from build123d import *

# Parameters (mm, degrees)
CROQUIS1_R              = 100
SALIENTE_EXTRUIR1_DEPTH = 3
CROQUIS3_R              = 110
CORTAR_EXTRUIR1_DEPTH   = 3
REDONDEO1_R             = 10
CORTAR_EXTRUIR2_DEPTH   = 142.453172607
CROQUIS6_W              = 10
CROQUIS6_H              = 50
CROQUIS6_W_2            = 30
CROQUIS6_H_2            = 10
CORTAR_EXTRUIR4_DEPTH   = 10
REDONDEO3_R             = 5
CROQUIS7_R              = 1.5
CORTAR_EXTRUIR5_DEPTH   = 142.453172607
CROQUIS8_R              = 1.5
CORTAR_EXTRUIR6_DEPTH   = 142.453172607
CROQUIS9_R              = 2
CORTAR_EXTRUIR7_DEPTH   = 142.453172607


with BuildPart() as part:
    # Croquis1 → Saliente-Extruir1 (new body)
    with BuildSketch(Plane.XY):
        Circle(CROQUIS1_R)
    extrude(amount=SALIENTE_EXTRUIR1_DEPTH)

    # Croquis3 → Cortar-Extruir1 (cut)
    with BuildSketch(Plane.XY.offset(3)):
        with Locations((190, 0)):
            Circle(CROQUIS3_R)
    extrude(amount=-CORTAR_EXTRUIR1_DEPTH, mode=Mode.SUBTRACT)

    # Redondeo1
    redondeo1_edges = [part.edges().sort_by_distance(p)[0] for p in [
        (89.473684211, -44.659375654, 1.5),
        (89.473684211, 44.659375654, 1.5),
    ]]
    fillet(redondeo1_edges, radius=REDONDEO1_R)

    # Croquis4 → Cortar-Extruir2 (cut, through all)
    with BuildSketch(Plane.XY.offset(3)):
        Polygon((-57.629202667, -83.792153571), (-83.792153571, -57.629202667), (-68.235804385, -42.072853481), (-42.072853481, -68.235804385), align=None)
        Polygon((-57.629202667, 83.792153571), (-42.072853481, 68.235804385), (-68.235804385, 42.072853481), (-83.792153571, 57.629202667), align=None)
        Polygon((83.792153571, 57.629202667), (68.235804385, 42.072853481), (42.072853481, 68.235804385), (57.629202667, 83.792153571), align=None)
        Polygon((57.629202667, -83.792153571), (42.072853481, -68.235804385), (68.235804385, -42.072853481), (83.792153571, -57.629202667), align=None)
    extrude(amount=-CORTAR_EXTRUIR2_DEPTH, mode=Mode.SUBTRACT)

    # Croquis6 → Cortar-Extruir4 (cut)
    with BuildSketch(Plane.XY.offset(3)):
        with Locations((-68.235804385, 0)):
            Rectangle(CROQUIS6_W, CROQUIS6_H)
        with Locations((0, 73.24)):
            Rectangle(CROQUIS6_W_2, CROQUIS6_H_2)
        with Locations((0, -73.24)):
            Rectangle(CROQUIS6_W_2, CROQUIS6_H_2)
    extrude(amount=-CORTAR_EXTRUIR4_DEPTH, mode=Mode.SUBTRACT)

    # Redondeo3
    redondeo3_edges = [part.edges().sort_by_distance(p)[0] for p in [
        (15, -78.24, 1.5),
        (-15, -78.24, 1.5),
        (15, -68.24, 1.5),
        (-15, -68.24, 1.5),
        (-73.235804385, -25, 1.5),
        (-63.235804385, -25, 1.5),
        (-73.235804385, 25, 1.5),
        (-63.235804385, 25, 1.5),
        (-15, 68.24, 1.5),
        (15, 68.24, 1.5),
        (-15, 78.24, 1.5),
        (15, 78.24, 1.5),
    ]]
    fillet(redondeo3_edges, radius=REDONDEO3_R - 0.0001)  # a hair under: the kernel refuses the full size

    # Croquis7 → Cortar-Extruir5 (cut, through all)
    with BuildSketch(Plane(origin=(0, 0, 0), x_dir=(-1, 0, 0), z_dir=(0, 0, -1))):
        with Locations((37.565, -24.17)):
            Circle(CROQUIS7_R)
        with Locations((-37.565, -24.17)):
            Circle(CROQUIS7_R)
        with Locations((-45.065, 24.17)):
            Circle(CROQUIS7_R)
        with Locations((37.565, 24.17)):
            Circle(CROQUIS7_R)
        with Locations((-14.06559482, 19.297497716)):
            Circle(CROQUIS7_R)
        with Locations((-14.061195262, -8.714642909)):
            Circle(CROQUIS7_R)
    extrude(amount=-CORTAR_EXTRUIR5_DEPTH, mode=Mode.SUBTRACT)

    # Croquis8 → Cortar-Extruir6 (cut, through all)
    with BuildSketch(Plane(origin=(0, 0, 0), x_dir=(-1, 0, 0), z_dir=(0, 0, -1))):
        with Locations((-20.32, 35)):
            Circle(CROQUIS8_R)
        with Locations((20.32, 35)):
            Circle(CROQUIS8_R)
        with Locations(Location((20.32, -35, 0), (0, 0, 180))):
            Circle(CROQUIS8_R)
        with Locations(Location((-20.32, -35, 0), (0, 0, 180))):
            Circle(CROQUIS8_R)
    extrude(amount=-CORTAR_EXTRUIR6_DEPTH, mode=Mode.SUBTRACT)

    # Croquis9 → Cortar-Extruir7 (cut, through all)
    with BuildSketch(Plane(origin=(0, 0, 0), x_dir=(-1, 0, 0), z_dir=(0, 0, -1))):
        with Locations((-35.206875778, 84.996916991)):
            Circle(CROQUIS9_R)
        with Locations((35.206875778, 84.996916991)):
            Circle(CROQUIS9_R)
        with Locations((84.996916991, 35.206875778)):
            Circle(CROQUIS9_R)
        with Locations((84.996916991, -35.206875778)):
            Circle(CROQUIS9_R)
        with Locations((35.206875778, -84.996916991)):
            Circle(CROQUIS9_R)
        with Locations((-35.206875778, -84.996916991)):
            Circle(CROQUIS9_R)
    extrude(amount=-CORTAR_EXTRUIR7_DEPTH, mode=Mode.SUBTRACT)


solid = part.part
CAD build for the part. Positions are in the model's coordinates, mm. A direction names the side the tool comes from. Round coordinates to 2 decimals unless told otherwise and drop trailing zeros. Loops run counter-clockwise (first coordinate to the right, second up) from the corner with the lowest first, then second, coordinate; pieces in that order, holes last. Notation, with made-up numbers: (-5.5, -36.5) - (6.5, -36.5) arc R20 cw to (6.5, -2.5) - close; hole circle Ø8 at (-12.5, -25). An arc over 180 degrees is marked (long way). Put each result on its own line as item: value.
1. Pin check, flat tips, straight feed: P1, Ø1.5, axis at y = -44, z = 1, coming from the -X side; P2, Ø1.8, axis at x = -37.565, y = -24.17, coming from the -Z side; P3, Ø1.5, axis at x = -48.5, z = 2.5, coming from the +Y side; P4, Ø1, axis at y = -22, z = 1.5, coming from the -X side. Stop position of each tip, or through.
Geometry check:
P1: x = -90.16
P2: through
P3: y = 87.86
P4: x = -97.66
2. 3-axis set-ups, long thin cutter, end or side, ignore diameter. For faces 4 (the cylindrical face through (-13.5, 69.67, 1.48)), 5 (the flat face through (49.14, 75.303, 1.521)), 6 (the flat face through (-49.341, 75.504, 1.521)), 7 (the flat face through (75.504, 49.341, 1.521)): which of +Z, -Z, +X, -X, +Y, -Y reach the whole face in a straight line?
Geometry check:
face 4: +Z, -Z
face 5: +Z, -Z, +X
face 6: +Z, -Z, -X
face 7: +Z, -Z, +Y
3. Slice it at B-B on y = 28.5. List the corners of the cut face in (x, z).
Geometry check:
outline: (-95.85, 0) - (83.76, 0) - (83.76, 3) - (-95.85, 3) - close
4. Wall check: line 1 (Y direction, x = -1, z = 2.25) (3 decimals); line 2 (Y direction, x = -34, z = 1.2); line 3 (X direction, y = -46.5, z = 2.05). Give the ranges that are in metal, low to high.
Geometry check:
line 1: -99.995 to -78.24, -68.24 to 68.24, 78.24 to 99.995
line 2: -94.04 to -86.59, -83.4 to 83.4, 86.59 to 94.04
line 3: -88.53 to -72.66, -63.81 to 63.81, 72.66 to 88.14
5. Two-plate mould, pull along Y, no slides. Class faces 1 (the cylindrical face through (-0.839, -99.996, 1.479)), 2 (the cylindrical face through (0.839, 99.996, 1.479)), 3 (the cylindrical face through (13.5, -76.81, 1.48)): released by +Y, released by -Y, zero draft, split by the parting line, or undercut.
Geometry check:
face 1: released by -Y
face 2: released by +Y
face 3: undercut
6. Slice it at A-A on z = 1.05. Give the number of separate pieces and of enclosed holes in the cut face, and give its area (3 significant figures).
Geometry check:
separate pieces: 1
enclosed holes: 19
area: 25,900 mm²
